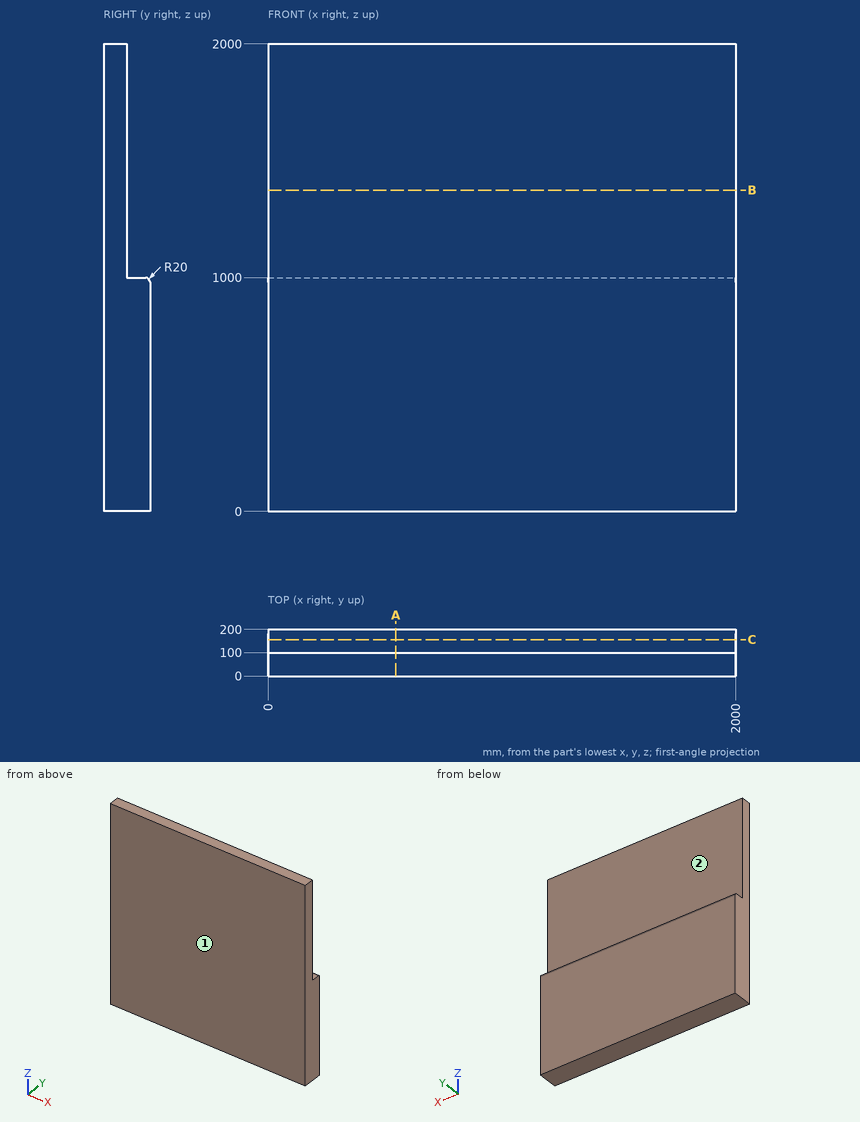
Print and shaded views of the part. All mm, measured from the part's lowest x, y and z. A direction names the side the tool comes from. Coordinates: 2 decimals unless noted, no trailing zeros. Order: outer loops, then holes, each group sorted by start corner. A loop starts at its lowest first (then second) coordinate and runs counter-clockwise, first axis right, second up. Notation, with made-up numbers: (63.5, 3) -> (90.5, 3) arc R28 cw to (90.5, 34) -> close; hole circle Ø9 at (84.25, 39). An arc over 180 degrees is marked (long way). Answer as a JSON object with one key per item and string values. Group by question number.
1) Drill centre lines: L1, parallel to Y at x = 253.5, z = 1703; L2, parallel to Z at x = 508.5, y = 181; L3, parallel to Z at x = 1141.5, y = 190. Where is each one in solid material? Low to high.
2) Cut at B-B, the plane z = 1374.5. Write the cut outline in (x, y).
3) Cut at C-C, the plane y = 156. Write the cut outline in (x, z).
4) Cut at A-A, the plane x = 546. Write the cut outline in (y, z), then the cut area to 3 significant figures.
5) Which spindle directions (+Z, -Z, +X, -X, +Y, -Y) get a long thin tool onto all of the face, cutting with end or side? Do the marked faces 1 and 2. Say none if no direction does.
Check values:
{
 "1": {"L1": "y = 0 to 100", "L2": "z = 0 to 999.97", "L3": "z = 0 to 997.32"},
 "2": {"outline": "(0, 0) -> (2000, 0) -> (2000, 100) -> (0, 100) -> close"},
 "3": {"outline": "(0, 0) -> (2000, 0) -> (2000, 1000) -> (0, 1000) -> close"},
 "4": {"outline": "(0, 0) -> (200, 0) -> (200, 980) arc R20 ccw to (180, 1000) -> (100, 1000) -> (100, 2000) -> (0, 2000) -> close", "area": "300,000 mm²"},
 "5": {"face 1": "+Z, -Z, +X, -X, -Y", "face 2": "+Z, +X, -X, +Y"}
}
